Input: part model. Units: mm. Frame: model coordinates. A direction names the side the tool comes from. Round coordinates to 2 decimals unless told otherwise and drop trailing zeros. Loops run counter-clockwise (first coordinate to the right, second up) from the corner with the lowest first, then second, coordinate; pieces in that order, holes last. Notation, with made-up numbers: (-21, 58.5) -> (38, 58.5) arc R27 cw to (38, 86.5) -> close; hole circle Ø7 at (73, -20.5). An arc over 180 degrees is marked (long way). Answer in a Markdown table with one row per item. Add a question column.
Q1. Mould query, pull axis Y, two halves, no side actions, for faces 1 (the face through (-1.75, 23.07, -44.36)), 2 (the face through (1.75, 26.533, -51.012)), 3 (the face through (-17.3, 47.1, 150)). Classes: pulls with the +Y half, pulls with the -Y half, needs draft (parallel to the pull), parting line crosses it, or undercut.
Q2. Section C-C, the plane x = 0. Output: boundary loops of the cut face in (y, z), and give its area (3 significant figures).
Q3. Section D-D, the plane z = 77. Output: boundary loops of the cut face in (x, y), and give its area (3 significant figures).
Q4. Reachability of faces 4 (the face through (53.115, -22.023, 90.617)), 5 (the face through (125, -17.3, 47.1)) from +Z, -Z, +X, -X, +Y, -Y: full face, straight path, thin tool, end or side. Return the list, or none.
Q5. Ray query, L1, parallel to X at y = 0, z = 77; L2, parallel to Z at x = -108.5, y = 1. Return the intervals inside material, ascending. Write a range as from..to.
Q6. Pin query (flat end, axial travel): pin 1 (1 mm diameter, centred on x = -84, y = -22, fed in from -Z); pin 2 (8 mm diameter, centred on x = -59.5, y = 24, fed in from -Z); pin 3 (6 mm diameter, centred on x = 79.5, y = 22, fed in from -Z). Return the tip coordinate at first contact, or that it passes through.
Q7. Section B-B, the plane z = 4. Output: boundary loops of the cut face in (x, y), and give its area (3 significant figures).
Q8. Section A-A, the plane y = 0. Output: boundary loops of the cut face in (x, z), and give its area (3 significant figures).
```python
from build123d import *

# Parameters (mm, degrees)
F0_R     = 57.5
F0_R_2   = 50
F1_DEPTH = 125
F2_R     = 57.5
F2_R_2   = 50
F3_DEPTH = 150
F4_R     = 50
F5_DEPTH = 250
F6_R     = 50
F7_DEPTH = 150


with BuildPart() as f1:
    # F0 (on Right) → F1 (new body, symmetric)
    with BuildSketch(Plane.YZ):
        Circle(F0_R)
        Circle(F0_R_2, mode=Mode.SUBTRACT)
    extrude(amount=F1_DEPTH, both=True)

    # F2 (on Top) → F3 (join)
    with BuildSketch(Plane.XY):
        Circle(F2_R)
        Circle(F2_R_2, mode=Mode.SUBTRACT)
    extrude(amount=F3_DEPTH)

    # F4 (on face) → F5 (cut)
    with BuildSketch(Plane(origin=(-125, 0, 0), x_dir=(0, -1, 0), z_dir=(-1, 0, 0))):
        Circle(F4_R)
    extrude(amount=-F5_DEPTH, mode=Mode.SUBTRACT)

    # F6 (on face) → F7 (cut)
    with BuildSketch(Plane.XY.offset(150)):
        Circle(F6_R)
    extrude(amount=-F7_DEPTH, mode=Mode.SUBTRACT)


solid = f1.part
```
Answer block:
| question | item | result |
|---|---|---|
| 1 | face 1 | undercut |
| 1 | face 2 | parting line crosses it |
| 1 | face 3 | needs draft |
| 2 | outline | (-57.5, 0) arc R57.5 ccw to (57.5, 0) -> (57.5, 150) -> (50, 150) -> (50, 0) arc R50 cw to (-50, 0) -> (-50, 150) -> (-57.5, 150) -> close |
| 2 | area | 3,520 mm^2 |
| 3 | outline | circle Ø115 at (0, 0); hole circle Ø100 at (0, 0) |
| 3 | area | 2,530 mm^2 |
| 4 | face 4 | +Z |
| 4 | face 5 | +Z, -Z, +X, +Y, -Y |
| 5 | L1 | -57.5..-50, 50..57.5 |
| 5 | L2 | -57.49..-49.99, 49.99..57.49 |
| 6 | pin 1 | z = -53.33 |
| 6 | pin 2 | z = -53.91 |
| 6 | pin 3 | z = -54.27 |
| 7 | outline | (-125, -57.36) -> (-4, -57.36) arc R57.5 ccw to (4, -57.36) -> (125, -57.36) -> (125, -49.84) -> (4, -49.84) arc R50 cw to (-4, -49.84) -> (-125, -49.84) -> close; (-125, 49.84) -> (-4, 49.84) arc R50 cw to (4, 49.84) -> (125, 49.84) -> (125, 57.36) -> (4, 57.36) arc R57.5 ccw to (-4, 57.36) -> (-125, 57.36) -> close |
| 7 | area | 3,760 mm^2 |
| 8 | outline | (-125, -57.5) -> (125, -57.5) -> (125, -50) -> (-125, -50) -> close; (-125, 50) -> (-50, 50) -> (-50, 150) -> (-57.5, 150) -> (-57.5, 57.5) -> (-125, 57.5) -> close; (50, 50) -> (125, 50) -> (125, 57.5) -> (57.5, 57.5) -> (57.5, 150) -> (50, 150) -> close |
| 8 | area | 4,390 mm^2 |
